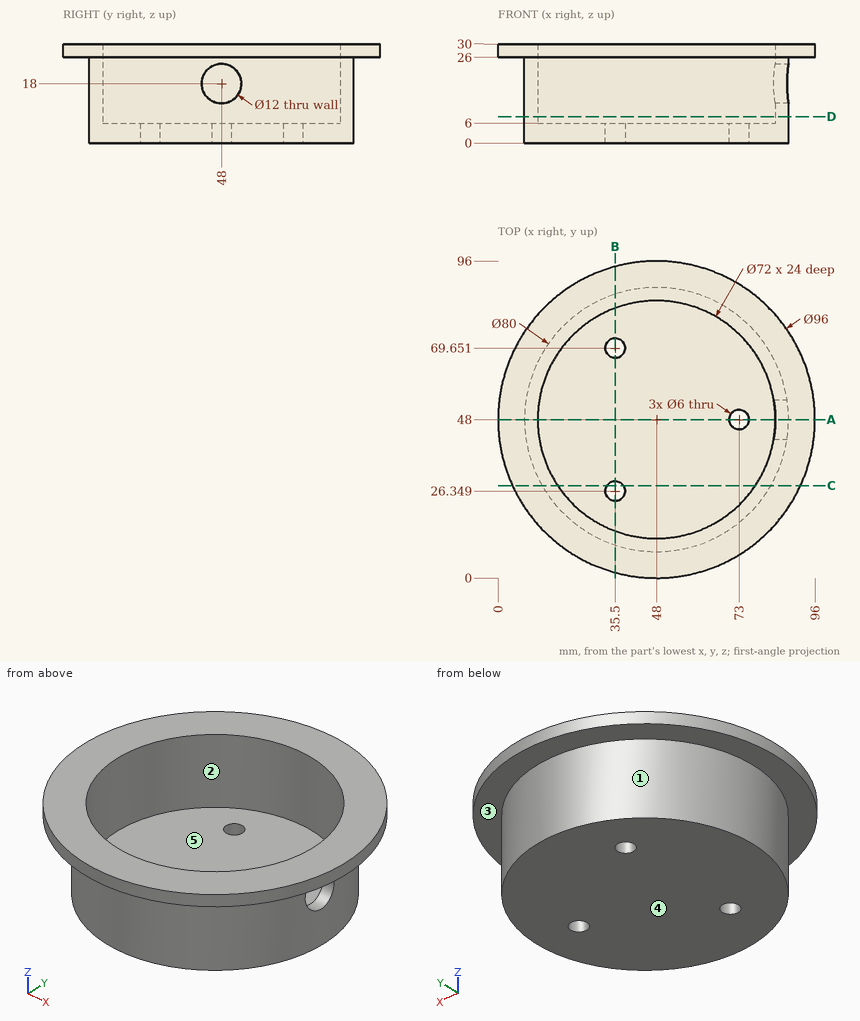
For this review, use the dimensioned drawing (mm, ordinates from the lowest corner) and the shaded views. A direction names the side the tool comes from. Give positions to 0.01 mm unless a question says otherwise; leave off trailing zeros. Write each loop counter-clockwise with the first axis right and the second up, starting at its lowest first coordinate (ties: lowest second). Pieces come first, ordered by that corner, then holes. Notation, with made-up numbers: M 30,68 L 42,68 A21 cw 42,91 Z; hole C 71,28 d11. An arc over 180 degrees is marked long. Answer as a JSON object with one key per item and string values. Group by question number.
1) We need section B-B (x = 35.5). Give the boundary of the cut face in (y, z).
2) Clearance check with flat-ended pins moving along their axes: pin 1 Ø5 at (x, y) = (35.5, 69.65) entering from -Z; pin 2 Ø10 at (x, z) = (39, 13) entering from -Y; pin 3 Ø12 at (x, y) = (27, 31) entering from +Z; pin 4 Ø1 at (x, z) = (27, 14.5) entering from +Y. State where each tip first meets the part, or that it passes through.
3) Mouldability with a two-part tool opening along X and no side actions: class the marked faces 1, 2 and 3 as released by +X, released by -X, zero draft, split by the parting line, or undercut.
4) We need section C-C (y = 28). Give the boundary of the cut face in (x, z) (1 decimal).
5) Tool access review of the marked faces 4 and 5: name each direction out of +Z, -Z, +X, -X, +Y, -Y from which nothing blocks a thin tool from reaching the whole face with its end or side.
6) We need section A-A (y = 48). Give the boundary of the cut face in (x, z).
7) For line 1 along Y through (x, z) = (35.5, 3.1); line 2 along Y through (x, z) = (48, 23); line 3 along Y through (x, z) = (57.5, 12) (1 decimal), list the stretches that pass through material, from the lowest coordinate up.
8) We need section D-D (z = 8). Give the boundary of the cut face in (x, y).
Answer key:
{
 "1": {"outline": "M 1.66,26 L 10,26 L 10,0 L 23.35,0 L 23.35,6 L 14.24,6 L 14.24,30 L 1.66,30 Z; M 29.35,0 L 66.65,0 L 66.65,6 L 29.35,6 Z; M 72.65,0 L 86,0 L 86,26 L 94.34,26 L 94.34,30 L 81.76,30 L 81.76,6 L 72.65,6 Z"},
 "2": {"pin 1": "passes through", "pin 2": "stops at y = 8.2", "pin 3": "stops at z = 6", "pin 4": "stops at y = 82.35"},
 "3": {"face 1": "split by the parting line", "face 2": "undercut", "face 3": "zero draft"},
 "4": {"outline": "M 4.4,26 L 13.4,26 L 13.4,0 L 33,0 L 33,6 L 18.1,6 L 18.1,30 L 4.4,30 Z; M 38,0 L 82.6,0 L 82.6,26 L 91.6,26 L 91.6,30 L 77.9,30 L 77.9,6 L 38,6 Z"},
 "5": {"face 4": "-Z, +X, -X, +Y, -Y", "face 5": "+Z"},
 "6": {"outline": "M 0,26 L 8,26 L 8,0 L 70,0 L 70,6 L 12,6 L 12,30 L 0,30 Z; M 76,0 L 88,0 L 88,12 L 84,12 L 84,6 L 76,6 Z; M 84,24 L 88,24 L 88,26 L 96,26 L 96,30 L 84,30 Z"},
 "7": {"line 1": "y = 10 to 23.35, 29.35 to 66.65, 72.65 to 86", "line 2": "y = 8 to 12, 84 to 88", "line 3": "y = 9.1 to 13.3, 82.7 to 86.9"},
 "8": {"outline": "C 48,48 d80; hole C 48,48 d72"}
}
